Source: CAD feature listing. Evaluate the final solid. Frame: model axes, mm. A direction names the side the tool comes from. Give positions to 0.01 mm unless a question says otherwise; leave off trailing zeros. Write each loop counter-clockwise with the first axis right and the second up, starting at its lowest first coordinate (ties: lowest second). Pieces come first, ordered by that corner, then holes.
```python
from build123d import *

# Parameters (mm, degrees)
SKETCH1_R           = 0.625
BOSS_EXTRUDE1_DEPTH = 4
SKETCH2_W           = 0.5
SKETCH2_H           = 2
SKETCH4_W           = 0.5
SKETCH4_H           = 2
BOSS_EXTRUDE2_DEPTH = 1.5


with BuildPart() as part:
    # Sketch1 → Boss-Extrude1 (new, symmetric)
    with BuildSketch(Plane(origin=(0, 0, 0), x_dir=(0, 0, -1), z_dir=(1, 0, 0))):
        Circle(SKETCH1_R)
    extrude(amount=BOSS_EXTRUDE1_DEPTH, both=True)

    # Sketch2 → Loft1 section 0
    with BuildSketch(Plane(origin=(5, 0, 0), x_dir=(0, 0, -1), z_dir=(1, 0, 0))):
        Rectangle(SKETCH2_W, SKETCH2_H)
    # Sketch3 for Loft1 → Loft1 section 1
    with BuildSketch(Plane(origin=(4, 0, 0), x_dir=(0, 0, -1), z_dir=(1, 0, 0))):
        with BuildLine():
            # circular arc as an exact rational Bezier (weights 1, cos(half-angle), 1)
            Bezier((0.151584766, -0.606339063), (0, -0.644235254), (-0.151584766, -0.606339063), weights=[1, 0.970142502, 1])
            Bezier((-0.151584766, -0.606339063), (-2.576941004, 0), (-0.151584766, 0.606339063), weights=[1, 0.242535626, 1])
            Bezier((-0.151584766, 0.606339063), (0, 0.644235254), (0.151584766, 0.606339063), weights=[1, 0.970142502, 1])
            Bezier((0.151584766, 0.606339063), (2.576941004, 0), (0.151584766, -0.606339063), weights=[1, 0.242535626, 1])
        make_face()
    loft1 = loft()

    # Sketch4 → Boss-Extrude2 (add)
    with BuildSketch(Plane(origin=(5, 0, 0), x_dir=(0, 0, -1), z_dir=(1, 0, 0))):
        Rectangle(SKETCH4_W, SKETCH4_H)
    boss_extrude2 = extrude(amount=BOSS_EXTRUDE2_DEPTH)

    # Mirror1: Loft1, Boss-Extrude2 across plane
    add(loft1.mirror(Plane(origin=(0, 0, 0), x_dir=(0, 0, 1), z_dir=(1, 0, 0))))
    add(boss_extrude2.mirror(Plane(origin=(0, 0, 0), x_dir=(0, 0, 1), z_dir=(1, 0, 0))))


solid = part.part
```
1. Line query: L1, parallel to Z at x = 5, y = 0.7; L2, parallel to Y at x = 2, z = 0.15. Output: solid intervals per line, ascending.
2. Contact query for flat-ended pins moving along their axis: P1, Ø1.2, axis at x = 6, y = -0.5, coming from the -Z side; P2, Ø1.2, axis at x = 6, y = 0.5, coming from the +Z side. Output: stop coordinate, or through.
3. Cut plane A-A, the plane x = 2. Return the cut outline in (y, z) (3 decimals), then the cut area to 3 significant figures.
4. Access query for faces 1 (the flat face through (6, 0, 0.25)), 2 (the cylindrical face through (0.06, -0.61, 0.14)), 3 (the flat face through (-6, 0, -0.25)), 4 (the flat face through (-6, 0, 0.25)), 5 (the flat face through (6, 0, -0.25)). Directions: +Z, -Z, +X, -X, +Y, -Y. A direction counts if a zero-diameter tool reaches every point of the face in a straight line with its end or side. Return the directions, or none.
Response values:
1. L1: z = -0.25 to 0.25
1. L2: y = -0.61 to 0.61
2. P1: stops at z = -0.25
2. P2: stops at z = 0.25
3. outline: circle Ø1.25 at (0, 0)
3. area: 1.23 mm2
4. face 1: +Z, +X, +Y, -Y
4. face 2: none
4. face 3: -Z, -X, +Y, -Y
4. face 4: +Z, -X, +Y, -Y
4. face 5: -Z, +X, +Y, -Y
